The drawing under review shows one solid part. Ordinate dimensions are in mm from its lowest x, y, z. Coordinates: 2 decimals unless noted, no trailing zeros. Loops run counter-clockwise (first coordinate to the right, second up) from the corner with the lowest first, then second, coordinate; pieces in that order, holes last.
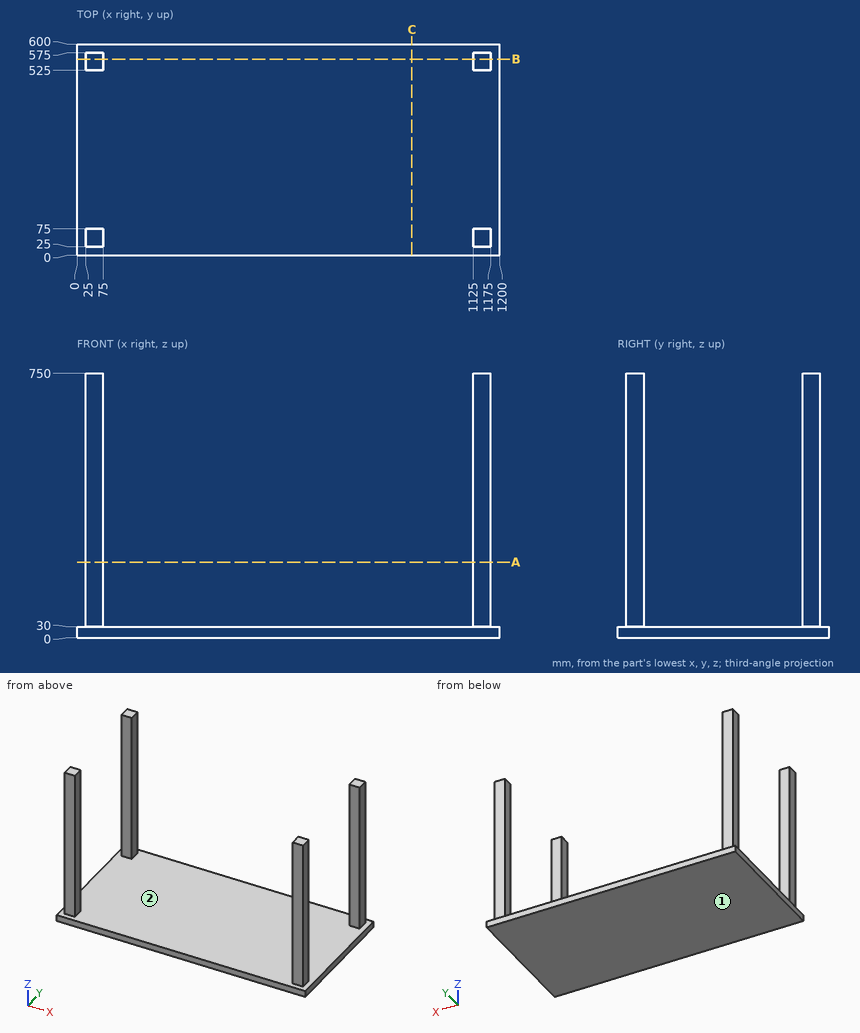
Q1. Take a section at B-B, the plane y = 557. Write out the cut boundary in (x, z).
Q2. Clearance check with flat-ended pins moving along their axes: pin 1 Ø2 at (x, y) = (351, 444) entering from +Z; pin 2 Ø25 at (x, z) = (51, 447.5) entering from -Y; pin 3 Ø1 at (x, y) = (423.5, 181) entering from -Z; pin 4 Ø25 at (y, z) = (559, 383.5) entering from -X. State where each tip first meets the part, or that it passes through.
Q3. Take a section at C-C, the plane x = 951. Write out the cut boundary in (y, z).
Q4. Take a section at A-A, the plane z = 214. Write out the cut boundary in (x, y), then the cut area to 3 significant figures.
Q5. The part is to be moulded in two halves that separate along X. For the marked faces 1 and 2, say which applies: pulls with the +X half, pulls with the -X half, needs draft (parallel to the pull), parting line crosses it, or undercut.
Q6. For line 1 (X direction, y = 534.5, z = 61.5); line 2 (Z direction, x = 483, y = 49), list the stretches that pass through material, from the lowest coordinate up.
Entries:
1. outline: (0, 0) - (1200, 0) - (1200, 30) - (1175, 30) - (1175, 750) - (1125, 750) - (1125, 30) - (75, 30) - (75, 750) - (25, 750) - (25, 30) - (0, 30) - close
2. pin 1: stops at z = 30
2. pin 2: stops at y = 25
2. pin 3: stops at z = 0
2. pin 4: stops at x = 25
3. outline: (0, 0) - (600, 0) - (600, 30) - (0, 30) - close
4. outline: (25, 25) - (75, 25) - (75, 75) - (25, 75) - close; (25, 525) - (75, 525) - (75, 575) - (25, 575) - close; (1125, 25) - (1175, 25) - (1175, 75) - (1125, 75) - close; (1125, 525) - (1175, 525) - (1175, 575) - (1125, 575) - close
4. area: 10,000 mm2
5. face 1: needs draft
5. face 2: undercut
6. line 1: x = 25 to 75, 1125 to 1175
6. line 2: z = 0 to 30
